Check sheet for the modelled part. Datum: model origin and axes. Units: mm. Coordinates: 2 decimals unless noted, no trailing zeros. Loops run counter-clockwise (first coordinate to the right, second up) from the corner with the lowest first, then second, coordinate; pieces in that order, holes last. Notation, with made-up numbers: (-29.75, 53.5) -> (23.25, 53.5) arc R22 ccw to (23.25, 68.5) -> close; hole circle Ø8 at (28, -27). An arc over 180 degrees is marked (long way). Use CSV: the item, a comma, the result in double quotes. Start each with the question number.
1. Release check for a two-part mould opening along Y. For faces 1 (the face through (0, -2, -2.5)), 2 (the face through (-6.944, -5.324, 0.035)), 3 (the face through (-0.195, 7.887, -0.035)) record: pulls with the +Y half, pulls with the -Y half, needs draft (parallel to the pull), parting line crosses it, or undercut.
2. Thickness scan on L1, parallel to Y at x = 0, z = -0.7; L2, parallel to X at y = -1, z = -2; L3, parallel to X at y = 0.25, z = -0.05. Record the ranges inside material, lowest first.
3. Sectioned sample at A-A, the plane x = 0. Record the cut outline in (y, z), and give its area (3 significant figures).
4. Gauge pin test, flat ends, axial feed: pin 1 (2 mm diameter, centred on x = 7, z = -1, fed in from +Y); pin 2 (3 mm diameter, centred on x = -4.5, z = -0.5, fed in from +Y); pin 3 (1 mm diameter, centred on y = -2.5, z = 0.5, fed in from -X). Record the tip position at first contact, or that the pin passes through.
5. Sectioned sample at B-B, the plane z = -0.1. Record the cut outline in (x, y).
6. Sectioned sample at C-C, the plane y = 6.4. Record the cut outline in (x, z).
```python
from build123d import *

# Parameters (mm, degrees)
SKETCH1_R           = 8.75
SKETCH1_R_2         = 1.5
EXTRUDE1_DEPTH      = 2.5
EXTRUDE2_DEPTH      = 13.624381173
EXTRUDE2_DEPTH_BACK = 13.624381173
SKETCH2_R           = 1.5


with BuildPart() as part:
    # Sketch1 → Extrude1 (new, symmetric)
    with BuildSketch(Plane.XY):
        Circle(SKETCH1_R)
        Circle(SKETCH1_R_2, mode=Mode.SUBTRACT)
    extrude(amount=EXTRUDE1_DEPTH, both=True)

    # Sketch2 → Extrude2 (cut, two sides: drawn at the far end of the back side and taken through both)
    with BuildSketch(Plane.XY.offset(-EXTRUDE2_DEPTH_BACK)):
        with Locations((0, 6.4)):
            Circle(SKETCH2_R)
        with Locations((6.4, 0)):
            Circle(SKETCH2_R)
        with Locations((0, -6.4)):
            Circle(SKETCH2_R)
        with Locations((-6.4, 0)):
            Circle(SKETCH2_R)
    extrude(amount=EXTRUDE2_DEPTH + EXTRUDE2_DEPTH_BACK, mode=Mode.SUBTRACT)


solid = part.part
```
Completed:
1,face 1,"needs draft"
1,face 2,"parting line crosses it"
1,face 3,"undercut"
2,L1,"-8.75 to -7.9, -4.9 to -1.5, 1.5 to 4.9, 7.9 to 8.75"
2,L2,"-8.69 to -7.52, -5.28 to -1.12, 1.12 to 5.28, 7.52 to 8.69"
2,L3,"-8.75 to -7.88, -4.92 to -1.48, 1.48 to 4.92, 7.88 to 8.75"
3,outline,"(-8.75, -2.5) -> (-7.9, -2.5) -> (-7.9, 2.5) -> (-8.75, 2.5) -> close; (-4.9, -2.5) -> (-1.5, -2.5) -> (-1.5, 2.5) -> (-4.9, 2.5) -> close; (1.5, -2.5) -> (4.9, -2.5) -> (4.9, 2.5) -> (1.5, 2.5) -> close; (7.9, -2.5) -> (8.75, -2.5) -> (8.75, 2.5) -> (7.9, 2.5) -> close"
3,area,"42.5 mm²"
4,pin 1,"y = 6.37"
4,pin 2,"y = 8.22"
4,pin 3,"x = -8.52"
5,outline,"circle Ø17.5 at (0, 0); hole circle Ø3 at (-6.4, 0); hole circle Ø3 at (0, -6.4); hole circle Ø3 at (0, 0); hole circle Ø3 at (0, 6.4); hole circle Ø3 at (6.4, 0)"
6,outline,"(-5.97, -2.5) -> (-1.5, -2.5) -> (-1.5, 2.5) -> (-5.97, 2.5) -> close; (1.5, -2.5) -> (5.97, -2.5) -> (5.97, 2.5) -> (1.5, 2.5) -> close"
